Design review of the part built by this model. Coordinates are the model's own, in mm. A direction names the side the tool comes from. Coordinates: 2 decimals unless noted, no trailing zeros. Write each loop counter-clockwise with the first axis right and the second up, starting at its lowest first coordinate (ties: lowest second). Pieces come first, ordered by that corner, then holes. Notation, with made-up numbers: (-2, 89.5) - (26, 89.5) arc R33 cw to (26, 128.5) - close; hole circle Ø7 at (79, -28.75). An arc over 180 degrees is marked (long way). Answer as CSV lines item,"result". Start each with the question number.
Q1. Mouldability with a two-part tool opening along Y and no side actions: class faces 6 (the face through (24.55, 1.72, 24.68)), 7 (the face through (-26, 7, 0)), 8 (the face through (11.34, -20.16, 24.68)) as pulls with the +Y half, pulls with the -Y half, needs draft (parallel to the pull), parting line crosses it, or undercut.
Q2. We need section D-D (x = 10). Write out the cut boundary in (y, z), plus the area to 3 significant figures.
Q3. For line 1 along Z through (x, y) = (1, -14); line 2 along Z through (x, y) = (-17, 0.5); line 3 along X through (y, z) = (-10.5, 38.5), list the stretches that pass through material, from the lowest coordinate up. Write a range as [from, to].
Q4. Machinability: for faces 1 (the face through (-26.898, 6.003, 25.35)), 2 (the face through (0, 2, -3)), 3 (the face through (0, -1, 2)), 4 (the face through (-24.53, 1.7, 24.68)), 5 (the face through (0, -2, -3)), which of the approach directions +Z, -Z, +X, -X, +Y, -Y give a long, thin tool a straight path to every point of the face, cutting with its end or side? Answer none if there is none.
Q5. We need section B-B (y = 7.5). Write out the cut boundary in (x, z), plus the area to 3 significant figures.
Q6. We need section C-C (z = 1). Write out the cut boundary in (x, y), plus the area to 3 significant figures.
Q7. We need section A-A (z = 40). Write out the cut boundary in (x, y), plus the area to 3 significant figures.
Q8. Clearance check with flat-ended pins moving along their axes: pin 1 (13 mm diameter, centred on y = -13, z = 24, fed in from +X); pin 2 (2 mm diameter, centred on y = 0, z = -4, fed in from +X); pin 3 (3 mm diameter, centred on x = -4.5, z = 8.5, fed in from -Y). State where each tip first meets the part, or that it passes through.
from build123d import *

# Parameters (mm, degrees)
EXTRUDE_1_DEPTH = 50
EXTRUDE_4_DEPTH = 50
SHELL_START     = 2
SHELL_1_DEPTH   = 46
SKETCH_4_W      = 55
SKETCH_4_H      = 18
EXTRUDE_5_DEPTH = 1
SKETCH_5_W      = 8
SKETCH_5_H      = 4
EXTRUDE_6_DEPTH = 5
FILLET_1_R      = 1


# Read off the part's stored shape, not the designer's step: 抽壳1
with BuildPart() as part:
    # 草图2 → 凸台-拉伸1 (new body)
    with BuildSketch(Plane.XY):
        Polygon((-25, -20), (0, -24), (25, -20), (25, 20), (-25, 20), align=None)
    extrude(amount=EXTRUDE_1_DEPTH)

    # 草图3 → 凸台-拉伸4 (add)
    with BuildSketch(Plane.XY):
        Polygon((-25, 5), (-27.5, 7.5), (-27.5, -6), (-25, -3.5), align=None)
        Polygon((27.5, -6), (25, -3.5), (25, 5), (27.5, 7.5), align=None)
    extrude(amount=EXTRUDE_4_DEPTH)

    # 抽壳1 outline → 抽壳1 (cut)
    with BuildSketch(Plane.XY.offset(SHELL_START)):
        Polygon((23, -18.294561776), (23, 20), (-23, 20), (-23, -18.294561776), (0, -21.974561776), align=None)
        Polygon((-25.5, -1.171572875), (-23.578427125, 0.75), (-25.5, 2.671572875), align=None)
        Polygon((23.578427125, 0.75), (25.5, -1.171572875), (25.5, 2.671572875), align=None)
    extrude(amount=SHELL_1_DEPTH, mode=Mode.SUBTRACT)

    # 草图4 → 凸台-拉伸5 (add)
    with BuildSketch(Plane(origin=(0, 0, 0), x_dir=(-1, 0, 0), z_dir=(0, 0, -1))):
        Rectangle(SKETCH_4_W, SKETCH_4_H)
    extrude(amount=EXTRUDE_5_DEPTH)

    # 草图5 → 凸台-拉伸6 (add)
    with BuildSketch(Plane.XY):
        Rectangle(SKETCH_5_W, SKETCH_5_H)
    extrude(amount=-EXTRUDE_6_DEPTH)

    # 圆角1
    fillet_1_edges = [part.edges().sort_by_distance(p)[0] for p in [
        (-27.5, 7.5, 25),
        (-27.5, -6, 25),
        (27.5, -6, 25),
        (27.5, 7.5, 25),
    ]]
    fillet(fillet_1_edges, radius=FILLET_1_R)


solid = part.part
Results list:
1,face 6,"undercut"
1,face 7,"needs draft"
1,face 8,"pulls with the +Y half"
2,outline,"(-22.4, 0) - (-9, 0) - (-9, -1) - (9, -1) - (9, 0) - (20, 0) - (20, 2) - (-20.37, 2) - (-20.37, 48) - (20, 48) - (20, 50) - (-22.4, 50) - close"
2,area,"281 mm2"
3,line 1,"z = [0, 2], [48, 50]"
3,line 2,"z = [-1, 2], [48, 50]"
3,line 3,"x = [-25, -23], [23, 25]"
4,face 1,"+Z, +Y"
4,face 2,"-Z, +X, -X, +Y"
4,face 3,"+Y"
4,face 4,"none"
4,face 5,"-Z, +X, -X, -Y"
5,outline,"(-27.5, -1) - (27.5, -1) - (27.5, 0) - (25, 0) - (25, 50) - (-25, 50) - (-25, 0) - (-27.5, 0) - close; hole (-23, 2) - (23, 2) - (23, 48) - (-23, 48) - close"
5,area,"439 mm2"
6,outline,"(-27.5, -3.59) arc R1 ccw to (-25.79, -4.29) - (-25, -3.5) - (-25, -20) - (0, -24) - (25, -20) - (25, -3.5) - (25.79, -4.29) arc R1 ccw to (27.5, -3.59) - (27.5, 5.09) arc R1 ccw to (25.79, 5.79) - (25, 5) - (25, 20) - (-25, 20) - (-25, 5) - (-25.79, 5.79) arc R1 ccw to (-27.5, 5.09) - close"
6,area,"2,150 mm2"
7,outline,"(-27.5, -3.59) arc R1 ccw to (-25.79, -4.29) - (-25, -3.5) - (-25, -20) - (0, -24) - (25, -20) - (25, -3.5) - (25.79, -4.29) arc R1 ccw to (27.5, -3.59) - (27.5, 5.09) arc R1 ccw to (25.79, 5.79) - (25, 5) - (25, 20) - (23, 20) - (23, -18.29) - (0, -21.97) - (-23, -18.29) - (-23, 20) - (-25, 20) - (-25, 5) - (-25.79, 5.79) arc R1 ccw to (-27.5, 5.09) - close; hole (-25.5, -1.17) - (-23.58, 0.75) - (-25.5, 2.67) - close; hole (23.58, 0.75) - (25.5, -1.17) - (25.5, 2.67) - close"
7,area,"296 mm2"
8,pin 1,"stops at x = 25"
8,pin 2,"stops at x = 4"
8,pin 3,"stops at y = -23.52"
